The model under review builds one solid part; all positions refer to its coordinate system, in mm. A direction names the side the tool comes from. Round coordinates to 2 decimals unless told otherwise and drop trailing zeros. Order: outer loops, then holes, each group sorted by start corner. A loop starts at its lowest first (then second) coordinate and runs counter-clockwise, first axis right, second up.
1) To check wall thickness, follow L1, parallel to Z at x = 0, y = 1.3; L2, parallel to Z at x = -0.5, y = 4.6; L3, parallel to X at y = 2.45, z = 28.5. State the ranges of each line that lie inside material, in increasing order.
2) Machinability: for faces 4 (the face through (-8, 2, -51)), 5 (the face through (-10, 2, 34)), 6 (the face through (10, 2, 34)), which of the approach directions +Z, -Z, +X, -X, +Y, -Y give a long, thin tool a straight path to every point of the face, cutting with its end or side? Answer none if there is none.
3) Mouldability with a two-part tool opening along X and no side actions: class faces 1 (the face through (10, 2, -30)), 2 (the face through (0.521, 2.465, 41.034)), 3 (the face through (-10, 2, -34)) as pulls with the +X half, pulls with the -X half, needs draft (parallel to the pull), parting line crosses it, or undercut.
4) Consider section B-B (y = 4). Give the boundary of the cut face in (x, z).
5) Consider section C-C (x = 20). Give the boundary of the cut face in (y, z).
6) Clearance check with flat-ended pins moving along their axes: P1, Ø2.5, axis at y = 2, z = 36.5, coming from the -X side; P2, Ø6, axis at x = 19.5, z = -51, coming from the -Y side; P3, Ø2, axis at x = 7.5, y = 3, coming from the -Z side; P4, Ø2, axis at y = 3.5, z = -41, coming from the +X side. State where each tip first meets the part, or that it passes through.
7) Consider section A-A (x = 0). Give the boundary of the cut face in (y, z), then the cut area to 3 significant figures.
8) Consider section D-D (z = 8). Give the boundary of the cut face in (x, y).
Autodesk Inventor part; units mm, degrees
ref_plane "YZ Plane" through (0, 0, 0) normal (1, 0, 0) x (0, 1, 0)
ref_plane "XZ Plane" through (0, 0, 0) normal (0, 1, 0) x (-1, 0, 0)
ref_plane "XY Plane" through (0, 0, 0) normal (0, 0, 1) x (1, 0, 0)
sketch "Sketch1" plane through (0, 0, 0) normal (0, 1, 0) x (-1, 0, 0)
  line L0 (0, 45) -> (0, -45) construction
  line L1 (-10, 45) -> (-10, -45)
  line L2 (10, -45) -> (10, 45)
  arc A0 (10, 45) -> (-10, 45) centre (0, 45) ccw
  arc A1 (-10, -45) -> (10, -45) centre (0, -45) ccw
  circle A2 centre (0, 45) radius 4
  circle A3 centre (0, -45) radius 4
  arc A4 (0, -45) -> (-64.2788, -121.6044) centre (25.1861, -131.404) ccw construction
  arc A5 (-2.7985, -35.3996) -> (-74.2193, -120.5156) centre (25.1861, -131.404) ccw
  arc A6 (2.7985, -54.6004) -> (-54.3382, -122.6933) centre (25.1861, -131.404) ccw
  arc A7 (2.7985, -54.6004) -> (-2.7985, -35.3996) centre (0, -45) ccw
  arc A8 (-74.2193, -120.5156) -> (-54.3382, -122.6933) centre (-64.2788, -121.6044) ccw
  line L3 (-64.2788, -121.6044) -> (0, -45)
  circle A9 centre (0, 0) radius 25
  point P0 (-6.4279, -52.6604)
  point P1 (10, -22.9129)
  point P2 (10, 22.9129)
  point P3 (-10, 22.9129)
  point P4 (-10, -22.9129)
  point P5 (-10, -37.7988)
  point P6 (-13.9586, -61.6352)
  point P7 (2.7985, -54.6004)
  dimension "d0" = 20
  dimension "d2" = 90
  dimension "d3" = 8
  dimension "d4" = 8
  dimension "d5" = 20
  dimension "d7" = 100
  dimension "d8" = 140
  dimension "d9" = 100
  dimension "d10" = 50
extrude "Extrusion1" add sketch "Sketch1" along normal blind 5 contours A0 L2 A9 L1 | A9 L2 L1 | L1 A9 | A9 L2 A7 A5 L1 | A9 L2 | A5 A7 A1 L1 | L1 A1 L3 A6 A8 A5 | A1 A6 L3
equation "\"d0\" = AnEsl"
equation "\"d5\" = AnEsl"
equation "\"d10\" = DV"
equation "\"DV\" = 50"
equation "\"AnEsl\" = 20"
properties part number "Pinzas"
Answer below:
1. L1: z = -55.47 to -49, -41 to 41, 49 to 55
1. L2: z = -55.31 to -48.97, -41.03 to 41.03, 48.97 to 54.99
1. L3: x = -10 to 10
2. face 4: -Z, -X, +Y, -Y
2. face 5: +Z, -X, +Y, -Y
2. face 6: +Z, +X, +Y, -Y
3. face 1: pulls with the +X half
3. face 2: undercut
3. face 3: pulls with the -X half
4. outline: (-10, -45) arc R10 ccw to (-2.8, -54.6) arc R80 cw to (54.34, -122.69) arc R10 ccw to (74.22, -120.52) arc R100 ccw to (10, -37.8) - (10, -22.91) arc R25 ccw to (10, 22.91) - (10, 45) arc R10 ccw to (-10, 45) - (-10, 22.91) arc R25 ccw to (-10, -22.91) - close; hole circle Ø8 at (0, -45); hole circle Ø8 at (0, 45)
5. outline: (0, -65.39) - (5, -65.39) - (5, -42.2) - (0, -42.2) - close; (0, -15) - (5, -15) - (5, 15) - (0, 15) - close
6. P1: stops at x = -10
6. P2: stops at y = 0
6. P3: stops at z = -58.84
6. P4: stops at x = 19.61
7. outline: (0, -55.47) - (5, -55.47) - (5, -49) - (0, -49) - close; (0, -41) - (5, -41) - (5, 41) - (0, 41) - close; (0, 49) - (5, 49) - (5, 55) - (0, 55) - close
7. area: 472 mm2
8. outline: (-23.69, 0) - (23.69, 0) - (23.69, 5) - (-23.69, 5) - close
